Check sheet for the modelled part. Datum: model origin and axes. Units: mm. Round coordinates to 2 decimals unless told otherwise and drop trailing zeros. Order: outer loops, then holes, each group sorted by start corner. A loop starts at its lowest first (then second) coordinate and runs counter-clockwise, first axis right, second up. Notation, with made-up numbers: M -6,12.5 L 36,12.5 A9 ccw 36,20.5 Z; hole C 25,70 d7. An arc over 180 degrees is marked long. One line per item, written item: value. Start each with the question number.
(1) Depth check by flat-ended pin: pin 1 Ø23 at (y, z) = (-769, 25.5) entering from -X; pin 2 Ø10 at (x, z) = (37.5, 44) entering from +Y; pin 3 Ø8 at (x, z) = (10, 42) entering from -Y. Enter the tip coordinate at first touch or a pass-through.
(2) Thickness scan on L1, parallel to X at y = -1130.5, z = 38. Record the ranges inside material, lowest first.
(3) Cross-section at C-C, the plane y = -1240.5. Enter the section's corners in (x, z), and give its area (3 significant figures).
(4) Cross-section at B-B, the plane z = 37. Enter the section's corners in (x, y), and give its area (3 significant figures).
(5) Cross-section at A-A, the plane x = 39.5. Enter the section's corners in (y, z).
from build123d import *

# Parameters (mm, degrees)
F0_W     = 50
F0_H     = 50
F0_W_2   = 46
F0_H_2   = 46
F1_DEPTH = 1600
F3_DEPTH = 50
F4_DEPTH = 50


with BuildPart() as f1:
    # F0 (on Front) → F1 (new body)
    with BuildSketch(Plane.XZ):
        with Locations((25, 25)):
            Rectangle(F0_W, F0_H)
        with Locations((25, 25)):
            Rectangle(F0_W_2, F0_H_2, mode=Mode.SUBTRACT)
    extrude(amount=F1_DEPTH)

    # F2 (on face) → F3 (cut)
    with BuildSketch(Plane.XY.offset(50)):
        Polygon((50, 0), (0, 0), (0, -50), align=None)
    extrude(amount=-F3_DEPTH, mode=Mode.SUBTRACT)

    # F2 (on face) → F4 (cut)
    with BuildSketch(Plane.XY.offset(50)):
        Polygon((50, 0), (0, 0), (0, -50), align=None)
        Polygon((0, -1550), (0, -1600), (50, -1600), align=None)
    extrude(amount=-F4_DEPTH, mode=Mode.SUBTRACT)


solid = f1.part
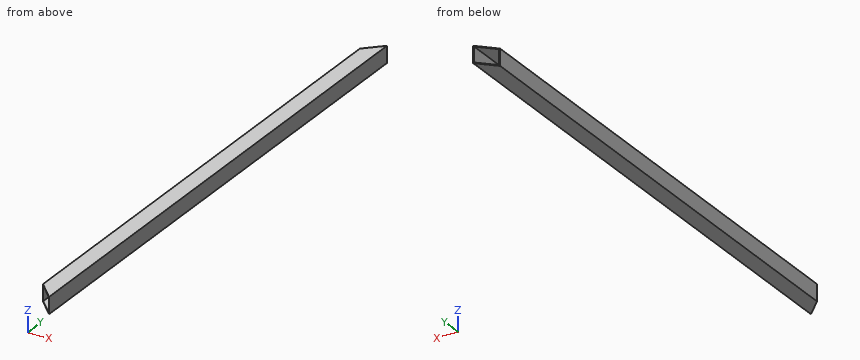
Values found:
1. pin 1: x = 0
1. pin 2: y = -9.5
1. pin 3: through
2. L1: 0 to 2, 48 to 50
3. outline: M 0,0 L 50,0 L 50,50 L 0,50 Z; hole M 2,2 L 48,2 L 48,48 L 2,48 Z
3. area: 384 mm^2
4. outline: M 0,-1550 L 2,-1552 L 2,-48 L 0,-50 Z; M 48,-1598 L 50,-1600 L 50,0 L 48,-2 Z
4. area: 6,200 mm^2
5. outline: M -1589.5,0 L -10.5,0 L -10.5,2 L -1589.5,2 Z; M -1589.5,48 L -10.5,48 L -10.5,50 L -1589.5,50 Z
